Can you work these out from the model? Positions are in its coordinate system, mm. A direction names the side the tool comes from. Coordinates: 2 decimals unless noted, no trailing zeros. Order: outer loops, then holes, each group sorted by start corner. A loop starts at its lowest first (then second) coordinate and runs counter-clockwise, first axis right, second up. Notation, with made-up numbers: (84.5, 60) -> (137.5, 60) arc R4 ccw to (137.5, 65) -> close; hole circle Ø10 at (64, -1). An arc over 180 degrees is marked (long way). Answer in a Markdown table with one row per item. Add a question column.
1. Imagine slicing it at C-C on y = 1.25. Write out the boundary of the cut face in (x, z).
2. We'd pull the mould along X, two halves only. Please class faces 5 (the face through (0, 0, 3)), 6 (the face through (-9.4, 7.5, -0.1)): pulls with the +X half, pulls with the -X half, needs draft (parallel to the pull), parting line crosses it, or undercut.
3. Imagine slicing it at A-A on x = 0. Write out the boundary of the cut face in (y, z), plus the area to 3 significant figures.
4. Imagine slicing it at B-B on z = 8. Write out the boundary of the cut face in (x, y).
5. Imagine slicing it at D-D on x = 3.5. Write out the boundary of the cut face in (y, z), plus the area to 3 significant figures.
6. If I drill on line 1 along X through (y, z) = (1.4, 0); line 2 along Z through (x, y) = (8, 2.5); line 3 along X through (y, z) = (1, 8), over which ranges is the centre line in solid material (lowest first)? Write a range as [from, to].
7. On a 3-axis mill with a long thin cutter (end or side, diameter ignored), from which of +Z, -Z, +X, -X, +Y, -Y can I reach the whole of each face in a straight line? I mean faces 1 (the face through (0, 8, 3)), 2 (the face through (9.59, 2.96, -9.5)), 3 (the face through (9.25, 5.04, 0.05)), 4 (the face through (-6.35, 1.01, -0.05)). Say none if no direction works.
8. Will these pins go through, and if not, where does the flat tip stop? pin 1 (4 mm diameter, centred on y = 4, z = 7, fed in from -X); pin 2 (0.6 mm diameter, centred on x = -7.5, y = 7.5, fed in from +Z); pin 3 (1.5 mm diameter, centred on y = 1, z = 8.5, fed in from +X).
from build123d import *

# Parameters (mm, degrees)
SKETCH_1_R               = 16.5
EXTRUDE_1_DEPTH          = 8
SKETCH_1_5_R             = 16.5
SKETCH_1_5_R_2           = 15.5
EXTRUDE_2_DEPTH          = 6
SKETCH_2_R               = 2.1
SKETCH_2_W               = 8.5
SKETCH_2_H               = 4.2
CUT_EXTRUDE_1_DEPTH      = 25.667792767
SKETCH_3_R               = 2.1
SKETCH_3_W               = 14.3
SKETCH_3_H               = 4.2
CUT_EXTRUDE_2_DEPTH      = 6
SKETCH_4_R               = 0.4
CUT_EXTRUDE_3_DEPTH      = 2
SKETCH_5_W               = 12.2
SKETCH_5_H               = 12.2
SKETCH_5_W_2             = 7
SKETCH_5_H_2             = 3.2
CUT_EXTRUDE_4_DEPTH      = 0.5
SKETCH_6_R               = 1
CUT_EXTRUDE_5_DEPTH      = 25.667792767
SKETCH_6_3_R             = 1.5
CUT_EXTRUDE_6_DEPTH      = 6
PATTERN_CIRCULAR_1_COUNT = 4


with BuildPart() as part:
    # 草图1 → 凸台-拉伸1 (new body)
    with BuildSketch(Plane(origin=(0, 0, 0), x_dir=(1, 0, 0), z_dir=(0, 1, 0))):
        with Locations(Location((0, 0, 0), (0, 0, 270))):
            Circle(SKETCH_1_R)
    extrude(amount=EXTRUDE_1_DEPTH)

    # 草图1<5> → 凸台-拉伸2 (add)
    with BuildSketch(Plane(origin=(0, 0, 0), x_dir=(1, 0, 0), z_dir=(0, 1, 0))):
        with Locations(Location((0, 0, 0), (0, 0, 270))):
            Circle(SKETCH_1_5_R)
        Circle(SKETCH_1_5_R_2, mode=Mode.SUBTRACT)
    extrude(amount=EXTRUDE_2_DEPTH)

    # 草图2 → 切除-拉伸1 (cut, through all)
    with BuildSketch(Plane(origin=(0, 8, 0), x_dir=(1, 0, 0), z_dir=(0, 1, 0))):
        with Locations((4.25, 0)):
            Circle(SKETCH_2_R)
        with Locations((-4.25, 0)):
            Circle(SKETCH_2_R)
        Rectangle(SKETCH_2_W, SKETCH_2_H)
    extrude(amount=-CUT_EXTRUDE_1_DEPTH, mode=Mode.SUBTRACT)

    # 草图3 → 切除-拉伸2 (cut)
    with BuildSketch(Plane(origin=(0, 8, 0), x_dir=(1, 0, 0), z_dir=(0, 1, 0))):
        with Locations((-7.15, 0)):
            Circle(SKETCH_3_R)
        with Locations((7.15, 0)):
            Circle(SKETCH_3_R)
        Rectangle(SKETCH_3_W, SKETCH_3_H)
    extrude(amount=-CUT_EXTRUDE_2_DEPTH, mode=Mode.SUBTRACT)

    # 草图4 → 切除-拉伸3 (cut)
    with BuildSketch(Plane(origin=(0, 2, 0), x_dir=(1, 0, 0), z_dir=(0, 1, 0))):
        with Locations(Location((-7.7, 0, 0), (0, 0, 270))):
            Circle(SKETCH_4_R)
        with Locations(Location((7.7, 0, 0), (0, 0, 270))):
            Circle(SKETCH_4_R)
    extrude(amount=-CUT_EXTRUDE_3_DEPTH, mode=Mode.SUBTRACT)

    # 草图5 → 切除-拉伸4 (cut)
    with BuildSketch(Plane(origin=(0, 8, 0), x_dir=(1, 0, 0), z_dir=(0, 1, 0))):
        with Locations((-8, 0)):
            Rectangle(SKETCH_5_W, SKETCH_5_H)
        with Locations((1.6, 0)):
            Rectangle(SKETCH_5_W_2, SKETCH_5_H_2)
    extrude(amount=-CUT_EXTRUDE_4_DEPTH, mode=Mode.SUBTRACT)

    # 草图6 → 切除-拉伸5 (cut, through all)
    with BuildSketch(Plane.XZ):
        with Locations(Location((8.485281374, 8.485281374, 0), (0, 0, 270))):
            Circle(SKETCH_6_R)
    cut_extrude_5 = extrude(amount=-CUT_EXTRUDE_5_DEPTH, mode=Mode.SUBTRACT)

    # 草图6<3> → 切除-拉伸6 (cut)
    with BuildSketch(Plane.XZ):
        with Locations(Location((8.485281374, 8.485281374, 0), (0, 0, 270))):
            Circle(SKETCH_6_3_R)
    cut_extrude_6 = extrude(amount=-CUT_EXTRUDE_6_DEPTH, mode=Mode.SUBTRACT)

    # 阵列(圆周)1: 切除-拉伸5, 切除-拉伸6 ×4 about axis
    pattern_circular_1_axis = Axis((0, 0, 0), (0, 1, 0))
    add([cut_extrude_5.rotate(pattern_circular_1_axis, i * 360 / PATTERN_CIRCULAR_1_COUNT) for i in range(1, PATTERN_CIRCULAR_1_COUNT)], mode=Mode.SUBTRACT)
    add([cut_extrude_6.rotate(pattern_circular_1_axis, i * 360 / PATTERN_CIRCULAR_1_COUNT) for i in range(1, PATTERN_CIRCULAR_1_COUNT)], mode=Mode.SUBTRACT)


solid = part.part
Answers follow:
| question | item | result |
|---|---|---|
| 1 | outline | circle Ø33 at (0, 0); hole circle Ø3 at (-8.49, -8.49); hole circle Ø3 at (-8.49, 8.49); hole circle Ø0.8 at (-7.7, 0); hole (-4.25, -2.1) -> (4.25, -2.1) arc R2.1 ccw to (4.25, 2.1) -> (-4.25, 2.1) arc R2.1 ccw to start; hole circle Ø3 at (8.49, -8.49); hole circle Ø3 at (8.49, 8.49); hole circle Ø0.8 at (7.7, 0) |
| 2 | face 5 | needs draft |
| 2 | face 6 | undercut |
| 3 | outline | (0, -16.5) -> (8, -16.5) -> (8, -2.1) -> (0, -2.1) -> close; (0, 2.1) -> (8, 2.1) -> (8, 16.5) -> (0, 16.5) -> close |
| 3 | area | 230 mm² |
| 4 | outline | (-14.43, 0) -> (-9.9, 0) -> (-9.9, 6) -> (-9.36, 6) -> (-9.36, 8) -> (-14.43, 8) -> close; (-7.61, 6) -> (-7.07, 6) -> (-7.07, 0) -> (7.07, 0) -> (7.07, 6) -> (7.61, 6) -> (7.61, 8) -> (-7.61, 8) -> close; (9.36, 6) -> (9.9, 6) -> (9.9, 0) -> (14.43, 0) -> (14.43, 8) -> (9.36, 8) -> close |
| 5 | outline | (0, -16.12) -> (8, -16.12) -> (8, -2.1) -> (0, -2.1) -> close; (0, 2.1) -> (8, 2.1) -> (8, 16.12) -> (0, 16.12) -> close |
| 5 | area | 224 mm² |
| 6 | line 1 | x = [-16.5, -8.1], [-7.3, -6.35], [6.35, 7.3], [8.1, 16.5] |
| 6 | line 2 | z = [-14.43, -9.9], [-7.07, -1.92], [1.92, 7.07], [9.9, 14.43] |
| 6 | line 3 | x = [-14.43, -9.9], [-7.07, 7.07], [9.9, 14.43] |
| 7 | face 1 | +Z, -Z, +X, -X, +Y |
| 7 | face 2 | -Y |
| 7 | face 3 | +Y |
| 7 | face 4 | +Y, -Y |
| 8 | pin 1 | stops at x = -15.72 |
| 8 | pin 2 | stops at z = 14.85 |
| 8 | pin 3 | stops at x = 14.57 |
